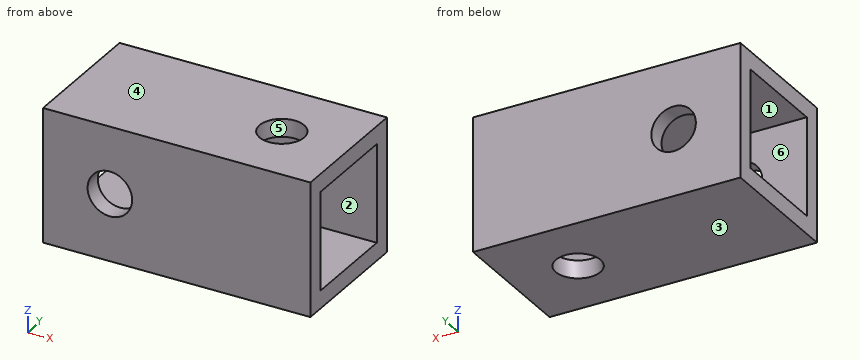
Autodesk Inventor part; units mm, degrees
ref_plane "YZ Plane" through (0, 0, 0) normal (1, 0, 0) x (0, 1, 0)
ref_plane "XZ Plane" through (0, 0, 0) normal (0, 1, 0) x (-1, 0, 0)
ref_plane "XY Plane" through (0, 0, 0) normal (0, 0, 1) x (1, 0, 0)
sketch "スケッチ1" plane through (0, 0, 0) normal (1, 0, 0) x (0, 1, 0)
  line L0 (0, 0) -> (9, 0)
  line L1 (9, 0) -> (9, -9)
  line L2 (9, -9) -> (0, -9)
  line L3 (0, -9) -> (0, 0)
  line L4 (1.2, -1.2) -> (7.8, -1.2)
  line L5 (7.8, -1.2) -> (7.8, -7.8)
  line L6 (7.8, -7.8) -> (1.2, -7.8)
  line L7 (1.2, -7.8) -> (1.2, -1.2)
  dimension "d0" = 9
  dimension "d1" = 9
  dimension "d3" = 1.2
  dimension "d5" = 1.2
  dimension "d6" = 1.2
  dimension "d7" = 1.2
extrude "押し出し1" add sketch "スケッチ1" along normal blind 18
sketch "スケッチ2" plane through (0, 9, 0) normal (0, 1, 0) x (1, 0, 0)
  line L0 (0, 9) -> (0, 0)
  line L1 (0, 9) -> (18, 9)
  point P0 (4.5, 4.5)
  dimension "d10" = 4.5
  dimension "d11" = 4.5
hole "穴1" at (4.5, 9, -4.5) direction (0, -1, 0) diameter 3 end through all
sketch "スケッチ3" plane through (0, 0, 0) normal (0, 0, 1) x (1, 0, 0)
  line L0 (0, 0) -> (18, 0)
  line L1 (0, 9) -> (0, 0)
  point P0 (13.5, 4.5)
  dimension "d19" = 4.5
  dimension "d20" = 13.5
hole "穴2" at (13.5, 4.5, 0) direction (0, 0, -1) diameter 3 end through all
equation "\"d5\" = d3"
equation "\"d6\" = d3"
equation "\"d7\" = d3"
properties part number "ロボット回転9x9x18" material "アルミニウム 6061"
Work out the finished part from the listing and answer in its coordinate system (mm). Face numbers are marked on the shaded views. A direction names the side the tool comes from. Round coordinates to 2 decimals unless told otherwise and drop trailing zeros. Order: outer loops, then holes, each group sorted by start corner. A loop starts at its lowest first (then second) coordinate and runs counter-clockwise, first axis right, second up. Notation, with made-up numbers: M 60,-11 L 98,-11 A10 ccw 98,1 Z; hole C 75,59 d10. An arc over 180 degrees is marked long. Put each result on its own line as item: value. Start each with the question number.
Q1. A tool of negligible diameter and unlimited length cuts with its end or side. For the marked faces 5 and 6, from which of +Z, -Z, +X, -X, +Y, -Y can it reach the whole face along a straight path? Write none if from no direction.
Q2. For a pull along Z with two mould halves and no side action, classify the marked faces 1, 2, 3 and 4 as pulls with the +Z half, pulls with the -Z half, needs draft (parallel to the pull), parting line crosses it, or undercut.
Q3. Straight lines are drawn through the part: L1, parallel to X at y = 4.5, z = -0.7; L2, parallel to Y at x = 15.5, z = -1.75; L3, parallel to Z at x = 10.5, y = 7. For each, find the intervals that lie inside material, in ascending order. Write a range as [from, to].
Q4. Section A-A, the plane z = -6.25 is taken. Write down the section's boundary in (x, y).
Q5. Section C-C, the plane y = 4.5 is taken. Write down the section's boundary in (x, z).
Q6. Section B-B, the plane x = 13.5 is taken. Write down the section's boundary in (y, z), and give its area (3 significant figures).
Q7. Section D-D, the plane z = -4.5 is taken. Write down the section's boundary in (x, y).
Findings below:
1. face 5: +Z, -Z
1. face 6: +X, -X
2. face 1: undercut
2. face 2: undercut
2. face 3: pulls with the -Z half
2. face 4: pulls with the +Z half
3. L1: x = [0, 12], [15, 18]
3. L2: y = [0, 1.2], [7.8, 9]
3. L3: z = [-9, -7.8], [-1.2, 0]
4. outline: M 0,0 L 18,0 L 18,1.2 L 0,1.2 Z; M 0,7.8 L 18,7.8 L 18,9 L 0,9 Z
5. outline: M 0,-9 L 12,-9 L 12,-7.8 L 0,-7.8 Z; M 0,-1.2 L 12,-1.2 L 12,0 L 0,0 Z; M 15,-9 L 18,-9 L 18,-7.8 L 15,-7.8 Z; M 15,-1.2 L 18,-1.2 L 18,0 L 15,0 Z
6. outline: M 0,-9 L 3,-9 L 3,-7.8 L 1.2,-7.8 L 1.2,-1.2 L 3,-1.2 L 3,0 L 0,0 Z; M 6,-9 L 9,-9 L 9,0 L 6,0 L 6,-1.2 L 7.8,-1.2 L 7.8,-7.8 L 6,-7.8 Z
6. area: 30.2 mm^2
7. outline: M 0,0 L 3,0 L 3,1.2 L 0,1.2 Z; M 0,7.8 L 3,7.8 L 3,9 L 0,9 Z; M 6,0 L 18,0 L 18,1.2 L 6,1.2 Z; M 6,7.8 L 18,7.8 L 18,9 L 6,9 Z
